Work out the finished part from the listing and answer in its coordinate system (mm). Give positions to 0.01 mm unless a question says otherwise; leave off trailing zeros. Loops run counter-clockwise (first coordinate to the right, second up) from the corner with the lowest first, then second, coordinate; pieces in that order, holes last. Notation, with made-up numbers: (67.25, 33.25) - (123.25, 33.25) arc R22 cw to (123.25, 49.25) - close; hole circle Ø3 at (-9.75, -23). An arc over 180 degrees is marked (long way). One line per question, with ' | ' between items. Start each with the question number.
1. For a pull along X with two mould halves and no side action, classify faces 1 (the face through (59.885, 4.227, -36.065)), 2 (the face through (-21.935, 4.696, -69.653)), 3 (the face through (15, 9.525, 1)) as released by +X, released by -X, zero draft, split by the parting line, or undercut.
2. Each of these flat-tipped pins is pushed along its axis until it touches: pin 1 (4.5 mm diameter, centred on x = 0, y = 4.76, fed in from +Z) (3 decimals); pin 2 (6 mm diameter, centred on x = 0, z = 57.531, fed in from -Y); pin 3 (0.8 mm diameter, centred on x = 0.5, y = 5, fed in from +Z) (3 decimals); pin 4 (4 mm diameter, centred on x = 45, y = 2.5, fed in from -Z). Where does it stop, or does it pass through?
3. Section A-A (z = 0) is taken. Determine the outline of the cut face in (x, y) (3 decimals), plus the area to 3 significant figures.
4. Section B-B (x = 15) is taken. Determine the outline of the cut face in (y, z) (3 decimals).
5. Find the intervals of material crossed by line 1 (X direction, y = 5, z = 0) (3 decimals); line 2 (Y direction, x = 0, z = 71) (1 decimal); line 3 (Z direction, x = 1.5, y = 7), in increasing order.
6. Section C-C (z = 43) is taken. Determine the outline of the cut face in (x, y) (3 decimals).
from build123d import *

# Parameters (mm, degrees)
SKETCH1_R               = 73.025
SKETCH1_R_2             = 3.2639
BOSS_EXTRUDE1_DEPTH     = 9.525
SKETCH4_R               = 1.397
CUT_EXTRUDE1_DEPTH      = 6.35
CIRPATTERN1_COUNT       = 3
CUT_EXTRUDE2_DEPTH      = 104.711267016
CUT_EXTRUDE2_DEPTH_BACK = 104.711267016
SKETCH5_R               = 1.5875


with BuildPart() as part:
    # Sketch1 → Boss-Extrude1 (new body)
    with BuildSketch(Plane(origin=(0, 0, 0), x_dir=(1, 0, 0), z_dir=(0, 1, 0))):
        with Locations(Location((0, 0, 0), (0, 0, 90))):
            Circle(SKETCH1_R)
        with Locations(Location((-49.823307505, 28.7655, 0), (0, 0, 90))):
            Circle(SKETCH1_R_2, mode=Mode.SUBTRACT)
        with Locations(Location((49.823307505, 28.7655, 0), (0, 0, 90))):
            Circle(SKETCH1_R_2, mode=Mode.SUBTRACT)
        with Locations(Location((0, -57.531, 0), (0, 0, 90))):
            Circle(SKETCH1_R_2, mode=Mode.SUBTRACT)
        with Locations(Location((0, 0, 0), (0, 0, 90))):
            Circle(SKETCH1_R_2, mode=Mode.SUBTRACT)
    extrude(amount=BOSS_EXTRUDE1_DEPTH)

    # Sketch4 → Cut-Extrude1 (cut)
    with BuildSketch(Plane.XY.offset(73.025)):
        with Locations((0, 4.7625)):
            Circle(SKETCH4_R)
    cut_extrude1 = extrude(amount=-CUT_EXTRUDE1_DEPTH, mode=Mode.SUBTRACT)

    # CirPattern1: Cut-Extrude1 ×3 about axis
    cirpattern1_axis = Axis((0, 0, 0), (0, 1, 0))
    for i in range(1, CIRPATTERN1_COUNT):
        add(cut_extrude1.rotate(cirpattern1_axis, i * 360 / CIRPATTERN1_COUNT), mode=Mode.SUBTRACT)

    # Sketch5 → Cut-Extrude2 (cut, two sides: drawn at the far end of the back side and taken through both)
    with BuildSketch(Plane(origin=(0, 9.525, 0), x_dir=(1, 0, 0), z_dir=(0, 1, 0)).offset(-CUT_EXTRUDE2_DEPTH_BACK)):
        with Locations(Location((3.918177901, 24.089251357, 0), (0, 0, 270))):
            Circle(SKETCH5_R)
    extrude(amount=CUT_EXTRUDE2_DEPTH + CUT_EXTRUDE2_DEPTH_BACK, mode=Mode.SUBTRACT)


solid = part.part
Conclusion:
1) face 1: undercut | face 2: split by the parting line | face 3: zero draft
2) pin 1: z = 73.025 | pin 2: through | pin 3: z = 66.675 | pin 4: z = -59.02
3) outline: (-73.025, 0) - (-3.264, 0) - (-3.264, 9.525) - (-73.025, 9.525) - close; (3.264, 0) - (73.025, 0) - (73.025, 9.525) - (3.264, 9.525) - close | area: 1,330 mm²
4) outline: (0, -71.468) - (9.525, -71.468) - (9.525, 71.468) - (0, 71.468) - close
5) line 1: -73.025 to -3.264, 3.264 to 73.025 | line 2: 0 to 3.4, 6.2 to 9.5 | line 3: -73.01 to -2.9, 2.9 to 54.63, 60.43 to 73.01
6) outline: (-59.022, 0) - (59.022, 0) - (59.022, 9.525) - (-59.022, 9.525) - close
